For this review, take the finished solid that the model builds, in its own axes (mm). A direction names the side the tool comes from. Give positions to 0.01 mm unless a question says otherwise; leave off trailing zeros. Order: outer loops, then holes, each group sorted by start corner. A loop starts at its lowest first (then second) coordinate and runs counter-clockwise, first axis right, second up. Notation, with made-up numbers: (76.5, -7.5) - (100.5, -7.5) arc R22 cw to (100.5, 29.5) - close; hole circle Ø3 at (-6, -39). An arc over 180 degrees is marked (long way). Use a Markdown table: item, result. Add a question column.
1) Machinability: for faces 1 (the face through (0.6, 9.63, -1.41)), 2 (the face through (24.43, 9.63, -15.74)), 3 (the face through (12, 9, -16.34)), 4 (the face through (12, 9, -0.84)), which of the approach directions +Z, -Z, +X, -X, +Y, -Y give a long, thin tool a straight path to every point of the face, cutting with its end or side? Answer none if there is none.
2) We need section C-C on x = 10. Write out the cut boundary in (y, z).
3) We need section B-B on z = -9.25. Write out the cut boundary in (x, y), then the cut area to 3 significant figures.
4) Wall thickness on L1, parallel to X at y = 17, z = -8.25; L2, parallel to Z at x = 17, y = 15; L3, parallel to Y at x = 23, z = -0.5: over which ranges is each line inside the solid? List them lowest first.
5) We need section A-A on y = 3.75. Write out the cut boundary in (x, z).
6) Clearance check with flat-ended pins moving along their axes: P1, Ø9, axis at y = 13, z = -7, coming from the +X side; P2, Ø4, axis at y = 5.5, z = -10.5, coming from the -X side; P3, Ø5.5, axis at x = 10.5, y = 10, coming from the -Z side. State where each tip first meets the part, or that it passes through.
```python
from build123d import *

# Parameters (mm, degrees)
JIG_SKETCH_W   = 25
JIG_SKETCH_H   = 15.5
INSERT_DEPTH   = 20
SKETCH1_3_W    = 30
SKETCH1_3_H    = 20
BASE_DEPTH     = 5
ROUND_EDGES_R  = 2
CHAMFER_2_SIZE = 1


with BuildPart() as part:
    # jig_sketch → insert (new body)
    with BuildSketch(Plane(origin=(0, 0, 0), x_dir=(1, 0, 0), z_dir=(0, 1, 0))):
        with Locations((12.5, 8.590078954)):
            Rectangle(JIG_SKETCH_W, JIG_SKETCH_H)
    extrude(amount=INSERT_DEPTH)

    # Sketch1<3> → base (add)
    with BuildSketch(Plane(origin=(0, 0, 0), x_dir=(1, 0, 0), z_dir=(0, 1, 0))):
        with Locations((12.5, 8.590078954)):
            Rectangle(SKETCH1_3_W, SKETCH1_3_H)
    extrude(amount=-BASE_DEPTH)

    # round_edges
    round_edges_edges = [part.edges().sort_by_distance(p)[0] for p in [
        (0, 10, -0.840078954),
        (0, 10, -16.340078954),
        (25, 10, -16.340078954),
        (25, 10, -0.840078954),
    ]]
    fillet(round_edges_edges, radius=ROUND_EDGES_R)

    # chamfer 2
    chamfer_2_edges = [part.edges().sort_by_distance(p)[0] for p in [
        (25, 20, -8.590078954),
        (12.5, 20, -0.840078954),
        (12.5, 20, -16.340078954),
        (0, 20, -8.590078954),
        (0.585786438, 20, -1.425865392),
        (0.585786438, 20, -15.754292517),
        (24.414213562, 20, -15.754292517),
        (24.414213562, 20, -1.425865392),
    ]]
    chamfer(chamfer_2_edges, length=CHAMFER_2_SIZE)


solid = part.part
```
Checked values:
| question | item | result |
|---|---|---|
| 1 | face 1 | +Z, -X, +Y |
| 1 | face 2 | -Z, +X, +Y |
| 1 | face 3 | -Z, +X, -X, +Y |
| 1 | face 4 | +Z, +X, -X, +Y |
| 2 | outline | (-5, -18.59) - (0, -18.59) - (0, -16.34) - (19, -16.34) - (20, -15.34) - (20, -1.84) - (19, -0.84) - (0, -0.84) - (0, 1.41) - (-5, 1.41) - close |
| 3 | outline | (-2.5, -5) - (27.5, -5) - (27.5, 0) - (25, 0) - (25, 19) - (24, 20) - (1, 20) - (0, 19) - (0, 0) - (-2.5, 0) - close |
| 3 | area | 649 mm² |
| 4 | L1 | 0 to 25 |
| 4 | L2 | -16.34 to -0.84 |
| 4 | L3 | -5 to 0 |
| 5 | outline | (0, -14.34) arc R2 ccw to (2, -16.34) - (23, -16.34) arc R2 ccw to (25, -14.34) - (25, -2.84) arc R2 ccw to (23, -0.84) - (2, -0.84) arc R2 ccw to (0, -2.84) - close |
| 6 | P1 | x = 25 |
| 6 | P2 | x = 0 |
| 6 | P3 | z = -16.34 |
